```python
from build123d import *

# Parameters (mm, degrees)
SKETCH1_R           = 3.67665
BOSS_EXTRUDE1_DEPTH = 4.33
SKETCH2_R           = 2.235
CUT_EXTRUDE1_DEPTH  = 2.81
SKETCH3_R           = 2.29
CUT_EXTRUDE2_DEPTH  = 0.92
SKETCH4_R           = 1.27
CUT_EXTRUDE3_DEPTH  = 7.218006951
BOSS_EXTRUDE2_START = -1.65
BOSS_EXTRUDE2_DEPTH = 1.65
FILLET1_R           = 2
SKETCH6_R           = 0.4
CUT_EXTRUDE4_DEPTH  = 17.917177076


with BuildPart() as part:
    # Sketch1 → Boss-Extrude1 (new body)
    with BuildSketch(Plane.XY):
        Circle(SKETCH1_R)
    extrude(amount=BOSS_EXTRUDE1_DEPTH)

    # Sketch2 → Cut-Extrude1 (cut)
    with BuildSketch(Plane(origin=(0, 0, 0), x_dir=(-1, 0, 0), z_dir=(0, 0, -1))):
        Circle(SKETCH2_R)
    extrude(amount=-CUT_EXTRUDE1_DEPTH, mode=Mode.SUBTRACT)

    # Sketch3 → Cut-Extrude2 (cut)
    with BuildSketch(Plane.XY.offset(4.33)):
        Circle(SKETCH3_R)
    extrude(amount=-CUT_EXTRUDE2_DEPTH, mode=Mode.SUBTRACT)

    # Sketch4 → Cut-Extrude3 (cut, through all)
    with BuildSketch(Plane.XY.offset(3.41)):
        Circle(SKETCH4_R)
    extrude(amount=-CUT_EXTRUDE3_DEPTH, mode=Mode.SUBTRACT)

    # Sketch5 → Boss-Extrude2 (add)
    with BuildSketch(Plane.XY.offset(4.33).offset(BOSS_EXTRUDE2_START)):
        with BuildLine():
            ThreePointArc((-2.406107899, -2.78), (-3.67665, 0), (-2.406107899, 2.78))
            Line((-2.406107899, 2.78), (-15.935, 2))
            Line((-15.935, 2), (-15.935, -2))
            Line((-15.935, -2), (-2.406107899, -2.78))
        make_face()
    extrude(amount=BOSS_EXTRUDE2_DEPTH)

    # Fillet1
    fillet1_edges = [part.edges().sort_by_distance(p)[0] for p in [
        (-15.935, -2, 3.505),
        (-15.935, 2, 3.505),
    ]]
    fillet(fillet1_edges, radius=FILLET1_R)

    # Sketch6 → Cut-Extrude4 (cut, through all)
    with BuildSketch(Plane.XY.offset(4.33)):
        with Locations((-14.735, 0)):
            Circle(SKETCH6_R)
        with Locations((-12.735, 0)):
            Circle(SKETCH6_R)
        with Locations((-10.735, 0)):
            Circle(SKETCH6_R)
        with Locations((-8.735, 0)):
            Circle(SKETCH6_R)
        with Locations((-6.735, 0)):
            Circle(SKETCH6_R)
        with Locations((-4.735, 0)):
            Circle(SKETCH6_R)
    extrude(amount=-CUT_EXTRUDE4_DEPTH, mode=Mode.SUBTRACT)


solid = part.part
```
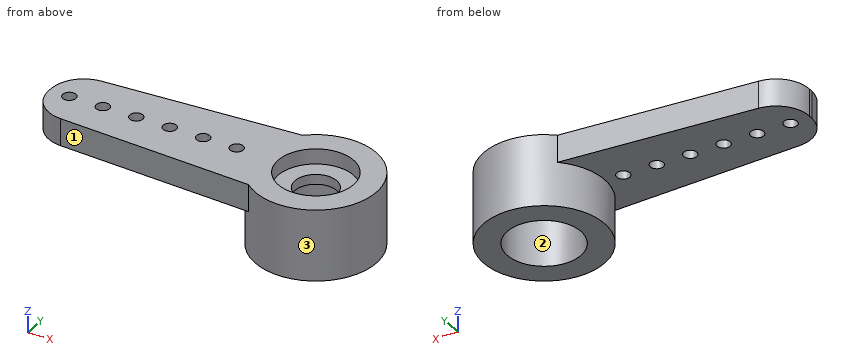
Can you work these out from the model? Positions are in its coordinate system, mm. Face numbers are marked on the shaded views. Round coordinates to 2 decimals unless told otherwise and drop trailing zeros. Loops run counter-clockwise (first coordinate to the right, second up) from the corner with the lowest first, then second, coordinate; pieces in that order, holes last. Notation, with made-up numbers: M 60,52 L 73,52 A17 ccw 73,62 Z; hole C -33.5,64 d6. An arc over 180 degrees is marked long. Answer in a Markdown table with one row per item.
1. I'm going to push flat-ended pins straight in: pin 1 Ø2.5 at (x, y) = (-1, 0.5) entering from +Z; pin 2 Ø3 at (x, y) = (-7, -1) entering from -Z; pin 3 Ø2 at (y, z) = (2.5, 1) entering from -X; pin 4 Ø4 at (x, y) = (0, 0) entering from +Z. Where does each tip first touch, or does it pass through?
Established:
| item | result |
|---|---|
| pin 1 | z = 4.33 |
| pin 2 | z = 2.68 |
| pin 3 | x = -3.36 |
| pin 4 | z = 3.41 |
2. If we section it at D-D, the plane z = 2.1: Please give me the cut outline in (x, y) (3 decimals), plus the area to 3 significant figures.
Established:
| item | result |
|---|---|
| outline | C 0,0 d7.353; hole C 0,0 d4.47 |
| area | 26.8 mm² |
3. If we section it at C-C, the plane y = -0.75: Please give me the cut outline in (x, z), plus the area to 3 significant figures.
Established:
| item | result |
|---|---|
| outline | M -15.83,2.68 L -3.6,2.68 L -3.6,0 L -2.11,0 L -2.11,2.81 L -1.02,2.81 L -1.02,3.41 L -2.16,3.41 L -2.16,4.33 L -15.83,4.33 Z; M 1.02,2.81 L 2.11,2.81 L 2.11,0 L 3.6,0 L 3.6,4.33 L 2.16,4.33 L 2.16,3.41 L 1.02,3.41 Z |
| area | 34.3 mm² |
4. Please list where these lines run through material, in increasing order: line 1 (Y direction, x = 0, z = 1.15) (3 decimals); line 2 (Y direction, x = -14.5, z = 4.1); line 3 (Z direction, x = -14.5, y = 0.5). Write a range as from..to.
Established:
| item | result |
|---|---|
| line 1 | -3.677..-2.235, 2.235..3.677 |
| line 2 | -2.03..-0.32, 0.32..2.03 |
| line 3 | 2.68..4.33 |
5. Thinking about a two-plate mould opening in X: for the marked faces 1, 2 and 3, which applies, pulls with the +X half, pulls with the -X half, needs draft (parallel to the pull), parting line crosses it, or undercut?
Established:
| item | result |
|---|---|
| face 1 | pulls with the -X half |
| face 2 | undercut |
| face 3 | parting line crosses it |
6. If we section it at B-B, the plane z = 4.1: Please give me the cut outline in (x, y) (3 decimals).
Established:
| item | result |
|---|---|
| outline | M -15.935,-0.112 A2 ccw -14.05,-2.109 L -2.406,-2.78 A3.677 ccw long -2.406,2.78 L -14.05,2.109 A2 ccw -15.935,0.112 Z; hole C -14.735,0 d0.8; hole C -12.735,0 d0.8; hole C -10.735,0 d0.8; hole C -8.735,0 d0.8; hole C -6.735,0 d0.8; hole C -4.735,0 d0.8; hole C 0,0 d4.58 |
7. If we section it at A-A, the plane x = 0: Please give me the cut outline in (y, z) (3 decimals), plus the area to 3 significant figures.
Established:
| item | result |
|---|---|
| outline | M -3.677,0 L -2.235,0 L -2.235,2.81 L -1.27,2.81 L -1.27,3.41 L -2.29,3.41 L -2.29,4.33 L -3.677,4.33 Z; M 1.27,2.81 L 2.235,2.81 L 2.235,0 L 3.677,0 L 3.677,4.33 L 2.29,4.33 L 2.29,3.41 L 1.27,3.41 Z |
| area | 13.5 mm² |
